The drawing under review shows one solid part. Ordinate dimensions are in mm from its lowest x, y, z. A direction names the side the tool comes from. Round coordinates to 2 decimals unless told otherwise and drop trailing zeros. Loops run counter-clockwise (first coordinate to the right, second up) from the corner with the lowest first, then second, coordinate; pieces in that order, holes last. Notation, with made-up numbers: (11.5, 42) - (58.5, 42) arc R27 cw to (58.5, 67) - close; hole circle Ø1 at (-5, -35.75). An arc over 180 degrees is marked (long way). Answer as CSV lines item,"result".
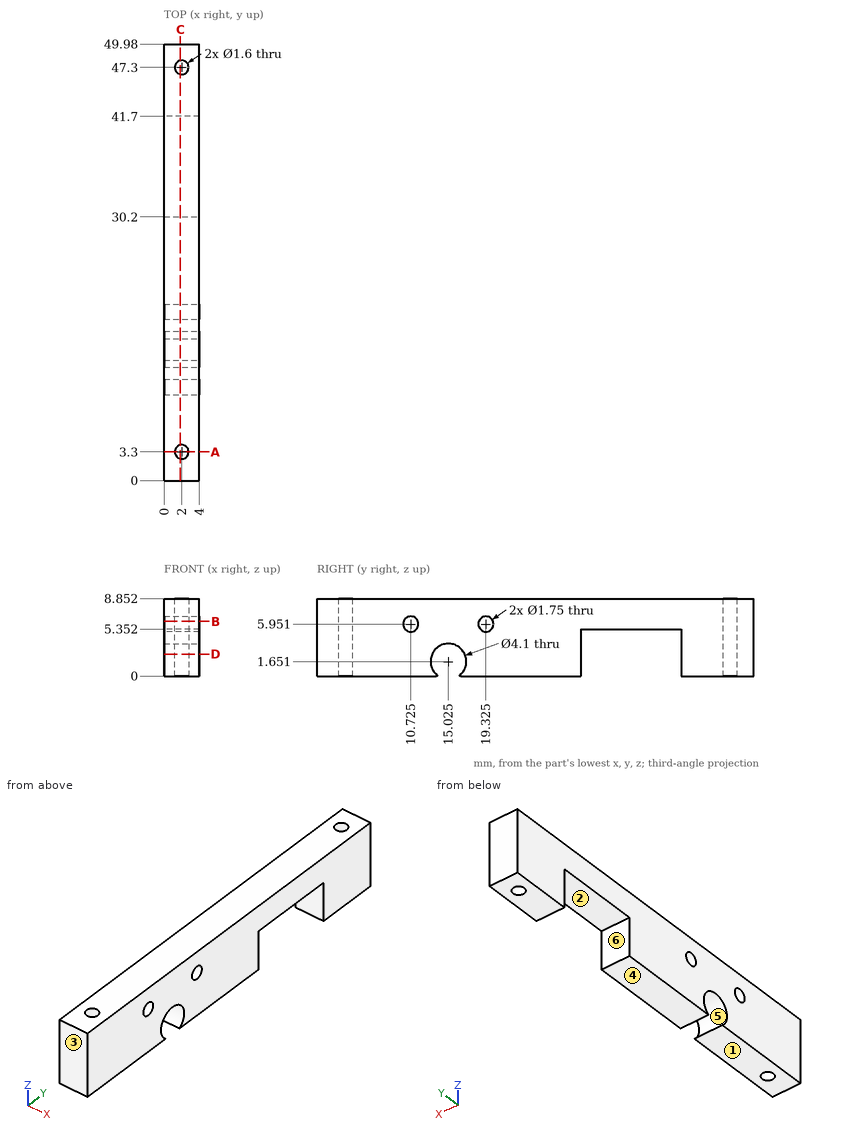
1. Draft analysis for pull direction Y (two halves, no side actions). For the marked faces 3, 4, 5 and 6, state which applies: +Y half, -Y half, draft (parallel to the pull), parting line (faces both ways), or undercut.
Numbers:
face 3,"-Y half"
face 4,"draft"
face 5,"undercut"
face 6,"undercut"
2. Take a section at C-C (x = 1.85). State how many separate pieces and enclosed holes the cut face has, plus the area to 3 significant figures.
Numbers:
separate pieces,"3"
enclosed holes,"2"
area,"336 mm²"
3. Wall thickness on probe 1 along Y at (x, z) = (2, 4.25); probe 2 along Y at (x, z) = (1.9, 6); probe 3 along Y at (x, z) = (0.6, 1.75): over which ranges is each line inside the solid? List them lowest first.
Numbers:
probe 1,"y = 0 to 2.5, 4.1 to 30.2, 41.7 to 46.5, 48.1 to 49.98"
probe 2,"y = 0 to 2.51, 4.09 to 9.85, 11.6 to 18.45, 20.2 to 46.51, 48.09 to 49.98"
probe 3,"y = 0 to 12.98, 17.07 to 30.2, 41.7 to 49.98"
4. Tool access review of the marked faces 1 and 2: name each direction out of +Z, -Z, +X, -X, +Y, -Y from which nothing blocks a thin tool from reaching the whole face with its end or side.
Numbers:
face 1,"-Z, +X, -X, +Y, -Y"
face 2,"-Z, +X, -X"
5. Take a section at B-B (z = 6.25). State the section outline as (x, y) points.
Numbers:
outline,"(0, 0) - (4, 0) - (4, 9.9) - (0, 9.9) - close; (0, 11.55) - (4, 11.55) - (4, 18.5) - (0, 18.5) - close; (0, 20.15) - (4, 20.15) - (4, 49.98) - (0, 49.98) - close; hole circle Ø1.6 at (2, 3.3); hole circle Ø1.6 at (2, 47.3)"
6. Take a section at A-A (y = 3.3). State the section outline as (x, z) points.
Numbers:
outline,"(0, 0) - (1.2, 0) - (1.2, 8.85) - (0, 8.85) - close; (2.8, 0) - (4, 0) - (4, 8.85) - (2.8, 8.85) - close"
7. Take a section at D-D (z = 2.5). State the section outline as (x, y) points, plus the area to 3 significant figures.
Numbers:
outline,"(0, 0) - (4, 0) - (4, 13.16) - (0, 13.16) - close; (0, 16.89) - (4, 16.89) - (4, 30.2) - (0, 30.2) - close; (0, 41.7) - (4, 41.7) - (4, 49.98) - (0, 49.98) - close; hole circle Ø1.6 at (2, 3.3); hole circle Ø1.6 at (2, 47.3)"
area,"135 mm²"
